For this review, take the finished solid that the model builds, in its own axes (mm). Face numbers are marked on the shaded views. A direction names the side the tool comes from. Give positions to 0.01 mm unless a question says otherwise; leave off trailing zeros. Write each loop counter-clockwise with the first axis right and the second up, starting at its lowest first coordinate (ties: lowest second). Pieces come first, ordered by that corner, then holes.
Q1. Insertion check: P1, Ø6, axis at x = 4.5, z = -7, coming from the +Y side; P2, Ø12.5, axis at x = 37, y = 13.5, coming from the +Z side; P3, Ø12, axis at x = 21, z = -22.5, coming from the -Y side; P4, Ø3, axis at y = 0.5, z = -8.5, coming from the -X side. Each pin has a flat end and moves straight along its axis. Give the tip position at first contact, or say it passes through.
Q2. We need section A-A (x = 53). Write out the cut boundary in (y, z).
Q3. Mouldability with a two-part tool opening along X and no side actions: class the marked faces 1, 2 and 3 as released by +X, released by -X, zero draft, split by the parting line, or undercut.
Q4. We need section D-D (x = 1). Write out the cut boundary in (y, z).
Q5. For line 1 (X direction, y = 19.1, z = -25); line 2 (X direction, y = 19.4, z = -25); line 3 (Z direction, x = 20, y = 5.25), list the stretches that pass through material, from the lowest coordinate up.
Q6. We need section C-C (z = -25). Write out the cut boundary in (x, y), then the cut area to 3 significant figures.
Q7. Machinability: for the marked faces 4 and 5, which of the approach directions +Z, -Z, +X, -X, +Y, -Y give a long, thin tool a straight path to every point of the face, cutting with its end or side? Answer none if there is none.
Q8. We need section B-B (y = -1). Write out the cut boundary in (x, z), then the cut area to 3 significant figures.
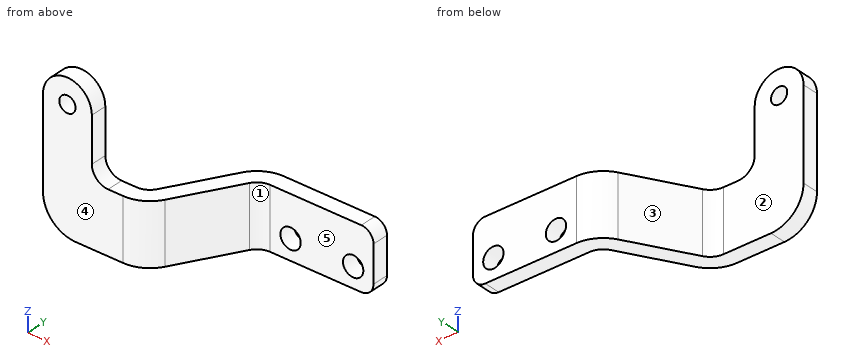
```python
from build123d import *

# Parameters (mm, degrees)
SKETCH_1_R                       = 2
SM_BASE_FLANGE_1_DEPTH           = 4
SM_EDGE_FLANGE_1_STRIP_CUT_DEPTH = 15
SM_EDGE_FLANGE_1_DEPTH           = 15
SM_EDGE_FLANGE_2_STRIP_CUT_DEPTH = 15
SM_EDGE_FLANGE_2_DEPTH           = 15
FILLET_1_R                       = 3
FILLET_2_R                       = 3
CUT_EXTRUDE_1_REACH              = 71.845
SKETCH_14_R                      = 2.5
CUT_EXTRUDE_1_DIRECTION_2_DEPTH  = 70.844662484


# Sheet-metal steps are written as plain solids
with BuildPart() as part:
    # Sketch 1 → Базовая кромка1 (new body)
    with BuildSketch(Plane(origin=(0, 0, 0), x_dir=(1, 0, 0), z_dir=(0, 1, 0))):
        with BuildLine():
            Line((-6, 0), (-6, 22))
            ThreePointArc((-6, 22), (-3.656854249, 27.656854249), (2, 30))
            Line((2, 30), (16, 30))
            Line((16, 30), (16, 15))
            Line((16, 15), (10, 15))
            ThreePointArc((10, 15), (7.171572875, 13.828427125), (6, 11))
            Line((6, 11), (6, 0))
            ThreePointArc((6, 0), (0, -6), (-6, 0))
        make_face()
        with Locations(Location((0, 0, 0), (0, 0, 270))):
            Circle(SKETCH_1_R, mode=Mode.SUBTRACT)
    extrude(amount=-SM_BASE_FLANGE_1_DEPTH)

    # Ребро-кромка1 strip (across the edge) → Ребро-кромка1 strip cut (cut)
    with BuildSketch(Plane(origin=(16, 0, -15), x_dir=(-0.8660254037844366, 0.5000000000000038, 0), z_dir=(0, 0, -1))):
        Polygon((-20.784609691, 7.381197846), (0, -4.618802154), (2, -1.154700538), (-18.784609691, 10.845299462), align=None)
    extrude(amount=SM_EDGE_FLANGE_1_STRIP_CUT_DEPTH, mode=Mode.SUBTRACT)

    # Ребро-кромка1 section (across the edge) → Ребро-кромка1 (add)
    with BuildSketch(Plane(origin=(16, 0, -15), x_dir=(-0.8660254037844366, 0.5000000000000038, 0), z_dir=(0, 0, -1))):
        with BuildLine():
            Line((-4, 2.309401077), (-4, 21.690598923))
            Line((-4, 21.690598923), (0, 21.690598923))
            Line((0, 21.690598923), (0, 2.309401077))
            ThreePointArc((0, 2.309401077), (0.535898385, 0.309401077), (2, -1.154700538))
            Line((2, -1.154700538), (0, -4.618802154))
            ThreePointArc((0, -4.618802154), (-2.92820323, -1.690598923), (-4, 2.309401077))
        make_face()
    extrude(amount=SM_EDGE_FLANGE_1_DEPTH)

    # Ребро-кромка2 strip (across the edge) → Ребро-кромка2 strip cut (cut)
    with BuildSketch(Plane(origin=(30.309401077, 16.784609691, -30), x_dir=(0, -1, 0), z_dir=(0, 0, 1))):
        Polygon((-20.784609691, 7.381197846), (0, -4.618802154), (2, -1.154700538), (-18.784609691, 10.845299462), align=None)
    extrude(amount=SM_EDGE_FLANGE_2_STRIP_CUT_DEPTH, mode=Mode.SUBTRACT)

    # Ребро-кромка2 section (across the edge) → Ребро-кромка2 (add)
    with BuildSketch(Plane(origin=(30.309401077, 16.784609691, -30), x_dir=(0, -1, 0), z_dir=(0, 0, 1))):
        with BuildLine():
            Line((-4, 2.309401077), (-4, 27.690598923))
            Line((-4, 27.690598923), (0, 27.690598923))
            Line((0, 27.690598923), (0, 2.309401077))
            ThreePointArc((0, 2.309401077), (0.535898385, 0.309401077), (2, -1.154700538))
            Line((2, -1.154700538), (0, -4.618802154))
            ThreePointArc((0, -4.618802154), (-2.92820323, -1.690598923), (-4, 2.309401077))
        make_face()
    extrude(amount=SM_EDGE_FLANGE_2_DEPTH)

    # Скругление1
    fillet_1_edges = [part.edges().sort_by_distance(p)[0] for p in [
        (58, 18.784609691, -15),
    ]]
    fillet(fillet_1_edges, radius=FILLET_1_R)

    # Скругление2
    fillet_2_edges = [part.edges().sort_by_distance(p)[0] for p in [
        (58, 18.784609691, -30),
    ]]
    fillet(fillet_2_edges, radius=FILLET_2_R)

    # Эскиз14 → Вырез-Вытянуть1 (cut, up to next)
    with BuildSketch(Plane(origin=(0, 20.784609691, 0), x_dir=(1, 0, 0), z_dir=(0, 1, 0)), mode=Mode.PRIVATE) as cut_extrude_1_sk1:
        with Locations((53, 25)):
            Circle(SKETCH_14_R)
    cut_extrude_1_tool1 = extrude(cut_extrude_1_sk1.sketch, amount=-CUT_EXTRUDE_1_REACH, mode=Mode.PRIVATE) & part.part
    # Эскиз14 → Вырез-Вытянуть1 (cut, up to next)
    with BuildSketch(Plane(origin=(0, 20.784609691, 0), x_dir=(1, 0, 0), z_dir=(0, 1, 0)), mode=Mode.PRIVATE) as cut_extrude_1_sk2:
        with Locations((37.618802154, 25)):
            Circle(SKETCH_14_R)
    cut_extrude_1_tool2 = extrude(cut_extrude_1_sk2.sketch, amount=-CUT_EXTRUDE_1_REACH, mode=Mode.PRIVATE) & part.part
    add(cut_extrude_1_tool1.solids().sort_by_distance((53, 20.78461, -25))[0], mode=Mode.SUBTRACT)
    add(cut_extrude_1_tool2.solids().sort_by_distance((37.618802, 20.78461, -25))[0], mode=Mode.SUBTRACT)

    # Эскиз14 → Вырез-Вытянуть1 direction 2 (cut)
    with BuildSketch(Plane(origin=(0, 20.784609691, 0), x_dir=(1, 0, 0), z_dir=(0, 1, 0))):
        with Locations((53, 25)):
            Circle(SKETCH_14_R)
        with Locations((37.618802154, 25)):
            Circle(SKETCH_14_R)
    extrude(amount=CUT_EXTRUDE_1_DIRECTION_2_DEPTH, mode=Mode.SUBTRACT)


solid = part.part
```
Computed:
1. P1: stops at y = 0
1. P2: stops at z = -15
1. P3: stops at y = -3.89
1. P4: stops at x = -6
2. outline: (16.78, -30) - (20.78, -30) - (20.78, -27.5) - (16.78, -27.5) - close; (16.78, -22.5) - (20.78, -22.5) - (20.78, -15) - (16.78, -15) - close
3. face 1: released by +X
3. face 2: zero draft
3. face 3: released by -X
4. outline: (-4, -29.94) - (0, -29.94) - (0, -1.73) - (-4, -1.73) - close; (-4, 1.73) - (0, 1.73) - (0, 5.92) - (-4, 5.92) - close
5. line 1: x = 27.71 to 35.12, 40.12 to 50.5, 55.5 to 58
5. line 2: x = 28.12 to 35.12, 40.12 to 50.5, 55.5 to 58
5. line 3: z = -30 to -15
6. outline: (-5.42, -4) - (13.69, -4) arc R8 ccw to (20.62, 0) - (29.15, 14.78) arc R4 cw to (32.62, 16.78) - (35.12, 16.78) - (35.12, 20.78) - (32.62, 20.78) arc R8 ccw to (25.69, 16.78) - (17.15, 2) arc R4 cw to (13.69, 0) - (-5.42, 0) - close; (40.12, 16.78) - (50.5, 16.78) - (50.5, 20.78) - (40.12, 20.78) - close; (55.5, 16.78) - (58, 16.78) - (58, 20.78) - (55.5, 20.78) - close
6. area: 257 mm2
7. face 4: +Z, -Z, +X, -X, -Y
7. face 5: +Z, -Z, +X, -Y
8. outline: (-6, -22) arc R8 ccw to (2, -30) - (19.94, -30) - (19.94, -15) - (10, -15) arc R4 cw to (6, -11) - (6, 0) arc R6 ccw to (-6, 0) - close; hole circle Ø4 at (0, 0)
8. area: 603 mm2
